```python
from build123d import *

# Parameters (mm, degrees)
BOSS_EXTRUDE1_DEPTH      = 60
SKETCH25_W               = 5.5
SKETCH25_H               = 17
BOSS_EXTRUDE3_DEPTH      = 20
FILLET1_R                = 2.3
SKETCH28_W               = 8
SKETCH28_H               = 10
CUT_EXTRUDE17_DEPTH      = 265
CUT_EXTRUDE19_DEPTH      = 165.638713704
CUT_EXTRUDE19_DEPTH_BACK = 165.638713704
SKETCH30_W               = 183.61
SKETCH30_H               = 30
CUT_EXTRUDE20_DEPTH      = 165.638713704
CUT_EXTRUDE20_DEPTH_BACK = 165.638713704
SKETCH32_W               = 3
SKETCH32_H               = 14
CUT_EXTRUDE23_DEPTH      = 44
CUT_EXTRUDE23_DEPTH_BACK = 254
SKETCH40_W               = 29.770973954
SKETCH40_H               = 62.053600945
SKETCH41_R               = 3
CUT_EXTRUDE24_DEPTH      = 254
BOSS_EXTRUDE4_DEPTH      = 40
CUT_EXTRUDE21_DEPTH      = 90
CUT_EXTRUDE22_DEPTH      = 164.320868502
CUT_EXTRUDE22_DEPTH_BACK = 164.320868502


with BuildPart() as part:
    # Sketch1 → Boss-Extrude1 (new body)
    with BuildSketch(Plane(origin=(0, 0, 0), x_dir=(1, 0, 0), z_dir=(0, 1, 0))):
        with BuildLine():
            Line((91.805, -10), (90.252689849, -10))
            ThreePointArc((90.252689849, -10), (0, -90.805), (-90.252689849, -10))
            Line((-90.252689849, -10), (-91.805, -10))
            Line((-91.805, -10), (-91.805, 20))
            Line((-91.805, 20), (-76.805, 20))
            Line((-76.805, 20), (-76.805, 0))
            ThreePointArc((-76.805, 0), (0, -76.805), (76.805, 0))
            Line((76.805, 0), (76.805, 20))
            Line((76.805, 20), (91.805, 20))
            Line((91.805, 20), (91.805, -10))
        make_face()
    extrude(amount=-BOSS_EXTRUDE1_DEPTH)

    # Sketch25 → Boss-Extrude3 (add)
    with BuildSketch(Plane(origin=(0, -60, 0), x_dir=(-1, 0, 0), z_dir=(0, -1, 0))):
        with Locations((84.305, 5)):
            Rectangle(SKETCH25_W, SKETCH25_H)
        with Locations((-84.305, 5)):
            Rectangle(SKETCH25_W, SKETCH25_H)
    extrude(amount=BOSS_EXTRUDE3_DEPTH)

    # Fillet1
    fillet1_edges = [part.edges().sort_by_distance(p)[0] for p in [
        (84.305, -60, 3.5),
        (81.555, -60, -5),
        (87.055, -60, -5),
        (84.305, -60, -13.5),
        (-84.305, -60, 3.5),
        (-87.055, -60, -5),
        (-81.555, -60, -5),
        (-84.305, -60, -13.5),
    ]]
    fillet(fillet1_edges, radius=FILLET1_R)

    # Sketch28 → Cut-Extrude17 (cut)
    with BuildSketch(Plane(origin=(91.805, 0, 0), x_dir=(0, 0, -1), z_dir=(1, 0, 0))):
        with Locations((5, -42)):
            Rectangle(SKETCH28_W, SKETCH28_H)
    extrude(amount=-CUT_EXTRUDE17_DEPTH, mode=Mode.SUBTRACT)

    # Sketch30 → Cut-Extrude19 (cut, two sides: drawn at the far end of the back side and taken through both)
    with BuildSketch(Plane(origin=(0, 0, -20), x_dir=(-1, 0, 0), z_dir=(0, 0, -1)).offset(-CUT_EXTRUDE19_DEPTH_BACK)):
        with Locations((0, -15)):
            Rectangle(SKETCH30_W, SKETCH30_H)
    extrude(amount=CUT_EXTRUDE19_DEPTH + CUT_EXTRUDE19_DEPTH_BACK, mode=Mode.SUBTRACT)

    # Sketch32 → Cut-Extrude20 (cut, two sides: drawn at the far end of the back side and taken through both)
    with BuildSketch(Plane(origin=(0, 0, -20), x_dir=(-1, 0, 0), z_dir=(0, 0, -1)).offset(-CUT_EXTRUDE20_DEPTH_BACK)):
        with Locations((51.773928511, -44)):
            Rectangle(SKETCH32_W, SKETCH32_H)
        with Locations((-65.13523483, -44)):
            Rectangle(SKETCH32_W, SKETCH32_H)
        with Locations((-51.773928511, -44)):
            Rectangle(SKETCH32_W, SKETCH32_H)
        with Locations((65.13523483, -44)):
            Rectangle(SKETCH32_W, SKETCH32_H)
    extrude(amount=CUT_EXTRUDE20_DEPTH + CUT_EXTRUDE20_DEPTH_BACK, mode=Mode.SUBTRACT)

    # Sketch40 → Cut-Extrude23 (cut, two sides: drawn at the far end of the back side and taken through both)
    with BuildSketch(Plane.ZY.offset(87.055).offset(-CUT_EXTRUDE23_DEPTH_BACK)):
        with Locations((-5.114513023, -61.026800472)):
            Rectangle(SKETCH40_W, SKETCH40_H)
    extrude(amount=CUT_EXTRUDE23_DEPTH + CUT_EXTRUDE23_DEPTH_BACK, mode=Mode.SUBTRACT)

    # Sketch41 → Cut-Extrude24 (cut)
    with BuildSketch(Plane(origin=(0, 0, 9.770973954), x_dir=(-1, 0, 0), z_dir=(0, 0, -1))):
        with Locations((-83.992971555, -37.5)):
            Circle(SKETCH41_R)
        with Locations((-83.992971555, -52.5)):
            Circle(SKETCH41_R)
        with Locations((83.992971555, -52.5)):
            Circle(SKETCH41_R)
        with Locations((83.992971555, -37.5)):
            Circle(SKETCH41_R)
    extrude(amount=-CUT_EXTRUDE24_DEPTH, mode=Mode.SUBTRACT)

    # Sketch33 → Boss-Extrude4 (add)
    with BuildSketch(Plane(origin=(0, -60, 0), x_dir=(-1, 0, 0), z_dir=(0, -1, 0))):
        with BuildLine():
            Line((90.252689849, -10), (76.151218145, -10))
            ThreePointArc((76.151218145, -10), (71.169996018, -28.876282513), (61.590580503, -45.886909008))
            Line((61.590580503, -45.886909008), (73.898492454, -52.768938193))
            ThreePointArc((73.898492454, -52.768938193), (84.815671791, -32.432234638), (90.252689849, -10))
        make_face()
    extrude(amount=BOSS_EXTRUDE4_DEPTH)

    # Sketch37 → Cut-Extrude21 (cut)
    with BuildSketch(Plane(origin=(0, 0, 0), x_dir=(0, 0, -1), z_dir=(1, 0, 0))):
        with BuildLine():
            Line((-0.881303102, -100), (-23.690614963, -100))
            ThreePointArc((-23.690614963, -100), (-31.684760451, -85.14357588), (-45.886909008, -76.037606625))
            Line((-45.886909008, -76.037606625), (-45.886909008, -59.917167305))
            Line((-45.886909008, -59.917167305), (-66.948234535, -59.917167305))
            Line((-66.948234535, -59.917167305), (-63.746381293, -92.441906362))
            Line((-63.746381293, -92.441906362), (-47.571757556, -115.346464391))
            Line((-47.571757556, -115.346464391), (-8.086377987, -115.346464391))
            Line((-8.086377987, -115.346464391), (-0.881303102, -100))
        make_face()
    extrude(amount=-CUT_EXTRUDE21_DEPTH, mode=Mode.SUBTRACT)

    # Sketch38 → Cut-Extrude22 (cut, two sides: drawn at the far end of the back side and taken through both)
    with BuildSketch(Plane(origin=(0, 0, 0), x_dir=(0, 0, -1), z_dir=(1, 0, 0)).offset(-CUT_EXTRUDE22_DEPTH_BACK)):
        Polygon((20, -30), (-90.805, -30), (-90.805, -60), (-10, -60), (-10, -100), (20, -100), (20, -60), align=None)
    extrude(amount=CUT_EXTRUDE22_DEPTH + CUT_EXTRUDE22_DEPTH_BACK, mode=Mode.SUBTRACT)


solid = part.part
```
The listing builds one solid part. Answer for the finished solid, in the listing's coordinates (mm). Coordinates: 2 decimals unless noted, no trailing zeros. Loops run counter-clockwise (first coordinate to the right, second up) from the corner with the lowest first, then second, coordinate; pieces in that order, holes last. Notation, with made-up numbers: (38.25, 58.25) -> (55.25, 58.25) arc R24 cw to (55.25, 90.25) -> close; hole circle Ø9 at (57, 67). An arc over 180 degrees is marked (long way). Return JSON: item names as keys, results as strings. Group by question number.
(1) A cutting plane is placed at A-A on y = -63. Write down the section's boundary in (x, z) (3 decimals), and give its area (3 significant figures).
(2) Given pin 1 Ø8 at (x, z) = (-72.5, 18) entering from -Y; pin 2 Ø4 at (x, z) = (-77, 36.5) entering from -Y; pin 3 Ø10 at (x, z) = (-65.5, 25) entering from -Y; pin 4 Ø1.5 at (y, z) = (-91.5, 22) entering from +X, each flat-ended and moving along its own axis, determine where each tip first touches the part or whether it passes through.
(3) A cutting plane is placed at D-D on x = -74.25. Write down the section's boundary in (y, z).
(4) Find the intervals of material crossed by probe 1 along X at (y, z) = (-75.5, 37.5); probe 2 along X at (y, z) = (-65, 28.5); probe 3 along Y at (x, z) = (-70.5, 44), in increasing order. Write a range as from..to.
(5) A cutting plane is placed at C-C on z = 32.5. Write down the section's boundary in (x, y).
(6) A cutting plane is placed at B-B on x = -83.25. Write down the section's boundary in (y, z).
The answers:
{
 "1": {"outline": "(-90.253, 10) -> (-76.151, 10) arc R76.805 cw to (-61.591, 45.887) -> (-78.358, 45.887) arc R90.805 ccw to start", "area": "540 mm^2"},
 "2": {"pin 1": "stops at y = -100", "pin 2": "stops at y = -82.44", "pin 3": "passes through", "pin 4": "stops at x = -73.36"},
 "3": {"outline": "(-100, 19.65) -> (-60, 19.65) -> (-60, 45.89) -> (-76.04, 45.89) arc R33.63 cw to (-100, 23.69) -> close"},
 "4": {"probe 1": "x = -82.7..-67.03", "probe 2": "x = -86.22..-71.32", "probe 3": "y = -76.72..-60"},
 "5": {"outline": "(-84.79, -84.29) -> (-69.59, -84.29) -> (-69.59, -60) -> (-84.79, -60) -> close"},
 "6": {"outline": "(-100, 10) -> (-60, 10) -> (-60, 36.26) -> (-81.03, 36.26) arc R33.63 cw to (-100, 23.69) -> close"}
}
